The listing builds one solid part. Answer for the finished solid, in the listing's coordinates (mm). Round coordinates to 2 decimals unless told otherwise and drop trailing zeros. Order: outer loops, then holes, each group sorted by start corner. A loop starts at its lowest first (then second) coordinate and runs counter-clockwise, first axis right, second up. Notation, with made-up numbers: M -1.75,-26.5 L 55.25,-26.5 A25 cw 55.25,5.5 Z; hole C -8,-15 d7. An arc over 180 degrees is marked long. Write item = value, one per line. Start each with the question number.
(1) Straight lines are drawn through the part: probe 1 along Z at (x, y) = (69, 64.5); probe 2 along Y at (x, z) = (80.5, 1316); probe 3 along Z at (x, y) = (38, 208). For each, find the intervals that lie inside material, in ascending order. Write a range as from..to.
(2) A cutting plane is placed at A-A, the plane y = 17.5. Determine the outline of the cut face in (x, z).
(3) Each of these flat-tipped pins is pushed along its axis until it touches: pin 1 (12.5 mm diameter, centred on x = 48.5, z = 51, fed in from -Y); pin 2 (1 mm diameter, centred on x = 55, y = 182.5, fed in from -Z); pin 3 (1 mm diameter, centred on x = 75, y = 149.5, fed in from -Z). Where does it stop, or does it pass through?
(4) A cutting plane is placed at B-B, the plane x = 90. Determine the outline of the cut face in (y, z).
(5) A cutting plane is placed at C-C, the plane y = 196. Determine the outline of the cut face in (x, z), and give its area (3 significant figures).
Autodesk Inventor part; units mm, degrees
ref_plane "Work Plane2" through (25.4038, 0, 736.5962) normal (0, -1, 0) x (1, 0, 0)
ref_plane "YZ Plane" through (0, 0, 0) normal (1, 0, 0) x (0, 1, 0)
ref_plane "XZ Plane" through (0, 0, 0) normal (0, 1, 0) x (-1, 0, 0)
sketch "Sketch1" plane through (0, 0, 0) normal (0, 0, 1) x (1, 0, 0)
  line L0 (0, 0) -> (0, 228.6)
  line L1 (0, 228.6) -> (76.2, 228.6)
  line L2 (76.2, 228.6) -> (76.2, 219.2528)
  line L3 (76.2, 219.2528) -> (101.6, 219.2528)
  line L4 (101.6, 219.2528) -> (101.6, 0)
  line L5 (101.6, 0) -> (0, 0)
  dimension "d0" = 228.6
  dimension "d1" = 76.2
  dimension "d2" = 9.3472
  dimension "d3" = 25.4
extrude "Extrusion1" add sketch "Sketch1" along normal blind 1422.4
ref_plane "Work Plane2" through (25.4038, 0, 736.5962) normal (0, -1, 0) x (1, 0, 0)
sketch "Sketch7" plane through (25.4038, 0, 736.5962) normal (0, -1, 0) x (1, 0, 0)
  line L0 (76.1962, -634.9962) -> (50.7962, -660.3962)
  line L1 (50.7962, -660.3962) -> (-0.0038, -660.3962)
  line L2 (76.1962, -634.9962) -> (-25.4038, -736.5962)
  line L3 (76.1962, -736.5962) -> (76.1962, 584.2038)
  line L4 (-0.0038, -660.3962) -> (-0.0038, -711.1962)
  line L5 (-0.0038, -711.1962) -> (50.7962, -660.3962)
  dimension "d39" = 50.8
  dimension "d41" = 90
  dimension "d42" = 50.8
extrude "Extrusion5" cut sketch "Sketch7" against normal blind 181.1528
sketch "Sketch8" plane through (25.4, 0, 76.2) normal (0, -1, 0) x (1, 0, 0)
  line L0 (76.2, -76.2) -> (76.2, 1346.2)
  line L1 (76.2, 1244.6) -> (50.8, 1270)
  line L2 (50.8, 1270) -> (0, 1270)
  line L3 (0, 1270) -> (0, 1320.8)
  line L4 (0, 1320.8) -> (50.8, 1270)
  line L5 (-25.4, 1346.2) -> (76.2, 1244.6)
  point P0 (-25.4, -76.2)
  point P1 (76.2, 25.4)
  dimension "d48" = 90
  dimension "d49" = 50.8
extrude "Extrusion6" cut sketch "Sketch8" against normal blind 181.1528
chamfer "Chamfer6" distance 101.6 angle 45 1 edges at (101.6, 109.6264, 1422.4)
chamfer "Chamfer7" distance 101.6 angle 45 1 edges at (101.6, 109.6264, 0)
sketch "Sketch9" plane through (25.4, 181.1528, 76.2) normal (0, -1, 0) x (1, 0, 0)
  line L0 (32.8422, -17.9578) -> (7.4422, -17.9578)
  line L1 (7.4422, -17.9578) -> (7.4422, -43.3578)
  line L2 (32.8422, -17.9578) -> (7.4422, -43.3578)
  line L3 (-25.4, -76.2) -> (50.8, 0)
  line L4 (50.8, 0) -> (38.1019, -12.6981)
  line L5 (50.8, 1270) -> (76.2, 1244.6)
  line L6 (50.8, 1270) -> (38.1019, 1282.6981)
  line L7 (0, 1320.8) -> (50.8, 1270)
  line L8 (38.1019, 1282.6981) -> (12.7019, 1282.6981)
  line L9 (12.7019, 1282.6981) -> (12.7019, 1308.0981)
  line L10 (38.1019, 1282.6981) -> (12.7019, 1308.0981)
  dimension "d63" = 0
  dimension "d64" = 25.4
  dimension "d65" = 17.9578
  dimension "d66" = 17.9578
  dimension "d67" = 25.4
extrude "Extrusion7" cut sketch "Sketch9" against normal blind 3.175 contours L7 L8 L9
sketch "Sketch10" plane through (25.4038, 181.1528, 736.5962) normal (0, -1, 0) x (1, 0, 0)
  line L0 (76.1962, -634.9962) -> (50.7962, -660.3962)
  line L1 (50.7962, -660.3962) -> (38.0981, -673.0942)
  line L2 (38.0981, -673.0942) -> (12.6981, -673.0942)
  line L3 (12.6981, -673.0942) -> (12.6981, -698.4942)
  line L4 (38.0981, -673.0942) -> (12.6981, -698.4942)
  point P0 (-25.4038, -736.5962)
  dimension "d70" = 17.9578
  dimension "d71" = 25.4
  dimension "d72" = 25.4
extrude "Extrusion8" cut sketch "Sketch10" against normal blind 3.175
properties part number "SideLength" material "Wood (Birch)"
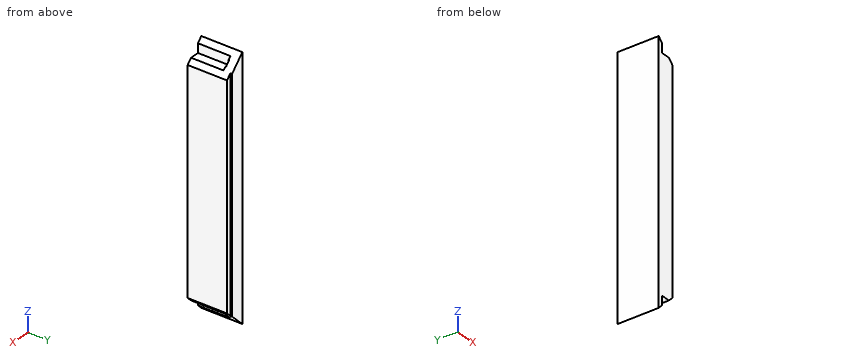
Reported:
q1.probe_1 = 76.2..1346.2
q1.probe_2 = 0..219.25
q1.probe_3 = 38..1384.4
q2.outline = M 0,0 L 25.4,25.4 L 25.4,76.2 L 76.2,76.2 L 101.6,101.6 L 101.6,1320.8 L 76.2,1346.2 L 25.4,1346.2 L 25.4,1397 L 0,1422.4 Z
q3.pin_1 = 184.33
q3.pin_2 = 63.5
q3.pin_3 = 76.2
q4.outline = M 0,90 L 219.25,90 L 219.25,1332.4 L 0,1332.4 Z
q5.outline = M 0,0 L 101.6,101.6 L 101.6,1320.8 L 0,1422.4 Z
q5.area = 134,000 mm²
